```python
from build123d import *

# Parameters (mm, degrees)
BOX002_W        = 24
BOX002_H        = 13.5
BOX002_DEPTH    = 8
SKETCH003_R     = 4.2
POCKET003_DEPTH = 14
SKETCH004_R     = 1.68
POCKET004_DEPTH = 8.001
FILLET_R        = 3


with BuildPart() as part:
    # Box002 → Box002 (new body)
    with BuildSketch(Plane(origin=(-2.5, 33, 0), x_dir=(1, 0, 0), z_dir=(0, 0, 1))):
        with Locations((12, 6.75)):
            Rectangle(BOX002_W, BOX002_H)
    extrude(amount=BOX002_DEPTH)

    # Sketch003 → Pocket003 (cut)
    with BuildSketch(Plane(origin=(-2.5, 46.5, 0), x_dir=(-1, 0, 0), z_dir=(0, 1, 0))):
        with Locations((-12, 8.3)):
            Circle(SKETCH003_R)
    extrude(amount=-POCKET003_DEPTH, mode=Mode.SUBTRACT)

    # Sketch004 → Pocket004 (cut, through all)
    with BuildSketch(Plane(origin=(-2.5, 33, 0), x_dir=(1, 0, 0), z_dir=(0, 0, -1))):
        with Locations((4, -7)):
            Circle(SKETCH004_R)
        with Locations((20, -7)):
            Circle(SKETCH004_R)
    extrude(amount=-POCKET004_DEPTH, mode=Mode.SUBTRACT)

    # Fillet
    fillet_edges = [part.edges().sort_by_distance(p)[0] for p in [
        (21.5, 33, 4),
        (-2.5, 33, 4),
    ]]
    fillet(fillet_edges, radius=FILLET_R)


solid = part.part
```
Model file for the job. Use its own axes, mm. Coordinates: 2 decimals unless noted, no trailing zeros. Order: outer loops, then holes, each group sorted by start corner. A loop starts at its lowest first (then second) coordinate and runs counter-clockwise, first axis right, second up. Notation, with made-up numbers: (-29.75, -6.75) -> (19.25, -6.75) arc R20 cw to (19.25, 18.25) -> close; hole circle Ø11 at (19.25, 7). An arc over 180 degrees is marked (long way). Return JSON: item names as keys, results as strings.
Item 1: Pin check, flat tip, straight feed: P1, Ø2.5, axis at x = 1.5, y = 40, coming from the +Z side. Stop position of the tip, or through.
Model answer:
{"P1": "passes through"}
Item 2: Slice it at D-D (z = 7). Write the cut outline in (x, y).
Model answer:
{"outline": "(-2.5, 36) arc R3 ccw to (0.5, 33) -> (5.51, 33) -> (5.51, 46.5) -> (-2.5, 46.5) -> close; (13.49, 33) -> (18.5, 33) arc R3 ccw to (21.5, 36) -> (21.5, 46.5) -> (13.49, 46.5) -> close; hole circle Ø3.36 at (1.5, 40); hole circle Ø3.36 at (17.5, 40)"}
Item 3: Slice it at A-A (z = 1.5). Write the cut outline in (x, y).
Model answer:
{"outline": "(-2.5, 36) arc R3 ccw to (0.5, 33) -> (18.5, 33) arc R3 ccw to (21.5, 36) -> (21.5, 46.5) -> (-2.5, 46.5) -> close; hole circle Ø3.36 at (1.5, 40); hole circle Ø3.36 at (17.5, 40)"}
Item 4: Mould opens along Y. For faces 1 (the face through (-1.64, 33.9, 4.06)), 2 (the face through (17.14, 41.64, 3.94)), 3 (the face through (1.14, 41.64, 3.94)), 4 (the face through (9, 40, 0)) say: pulls with the +Y half, pulls with the -Y half, needs draft (parallel to the pull), parting line crosses it, or undercut.
Model answer:
{"face 1": "pulls with the -Y half", "face 2": "undercut", "face 3": "undercut", "face 4": "needs draft"}
Item 5: Slice it at C-C (x = 1.5). Write the cut outline in (y, z).
Model answer:
{"outline": "(33, 0) -> (38.32, 0) -> (38.32, 8) -> (33, 8) -> close; (41.68, 0) -> (46.5, 0) -> (46.5, 8) -> (41.68, 8) -> close"}
Item 6: Slice it at B-B (y = 40). Write the cut outline in (x, z), then the cut area to 3 significant figures.
Model answer:
{"outline": "(-2.5, 0) -> (-0.18, 0) -> (-0.18, 8) -> (-2.5, 8) -> close; (3.18, 0) -> (15.82, 0) -> (15.82, 8) -> (13.69, 8) arc R4.2 cw to (5.31, 8) -> (3.18, 8) -> close; (19.18, 0) -> (21.5, 0) -> (21.5, 8) -> (19.18, 8) -> close", "area": "113 mm²"}
Item 7: Wall check: line 1 along Y through (x, z) = (17.5, 2.5); line 2 along X through (y, z) = (40.75, 7.5); line 3 along Y through (x, z) = (18.5, 2). Give the ranges that are in metal, low to high. Write a range as from..to.
Model answer:
{"line 1": "y = 33..38.32, 41.68..46.5", "line 2": "x = -2.5..0, 3..5.38, 13.62..16, 19..21.5", "line 3": "y = 33..38.65, 41.35..46.5"}
